Could you check a few things on this model? Use its own coordinates, in mm. A direction names the side the tool comes from. Round coordinates to 2 decimals unless told otherwise and drop trailing zeros. Write each loop counter-clockwise with the first axis right and the second up, starting at its lowest first coordinate (ties: lowest second). Pieces come first, ordered by that corner, then holes. Notation, with made-up numbers: (87.5, 9.25) -> (113.5, 9.25) arc R16 ccw to (113.5, 30.25) -> close; hole circle Ø8 at (67, -18). An arc over 180 degrees is marked (long way). Answer as CSV lines item,"result". Start each with the question number.
Q1. If we mould it in two halves opening along X, with no side actions, what happens to faces 1 (the flat face through (0, 6.1, -2)), 2 (the cylindrical face through (7.395, -2.028, 1.685)), 3 (the cylindrical face through (7.36, 1.99, -0.59))? For each: pulls with the +X half, pulls with the -X half, needs draft (parallel to the pull), parting line crosses it, or undercut.
Q2. For faces 4 (the flat face through (7.8, 3, -4.5)), 5 (the cylindrical face through (7.51, -2.03, 3.18)), 6 (the cylindrical face through (-4.956, 3.465, 5.072)), which set-ups out of +Z, -Z, +X, -X, +Y, -Y let a thin tool reach every point of the face, with its end or its side?
Q3. Imagine slicing it at B-B on y = -2.25. Please give me the cut outline in (x, z), and give its area (3 significant figures).
Q4. Imagine slicing it at D-D on x = 4.25. Please give me the cut outline in (y, z), and give its area (3 significant figures).
Q5. Imagine slicing it at C-C on y = 3.75. Please give me the cut outline in (x, z).
Q6. If I drill on line 1 (X direction, y = 0.6, z = -2.9); line 2 (Y direction, x = 4.5, z = 5.75); line 3 (Y direction, x = 5, z = -8), over which ranges is the centre line in solid material (lowest first)? Write a range as [from, to].
Q7. Will these pins go through, and if not, where does the flat tip stop? pin 1 Ø0.6 at (x, z) = (7.5, 3.5) entering from +Y; pin 2 Ø10 at (x, z) = (-4, 2) entering from -Y; pin 3 Ø1.6 at (x, z) = (-5, 6) entering from +Y.
Q8. Imagine slicing it at A-A on y = 1.5. Please give me the cut outline in (x, z).
from build123d import *

# Parameters (mm, degrees)
SKETCH1_W                = 17.5
SKETCH1_H                = 18
SKETCH1_R                = 0.4
BOSS_EXTRUDE1_DEPTH      = 1
SKETCH3_W                = 14
SKETCH3_H                = 17
SKETCH3_R                = 1
BOSS_EXTRUDE2_DEPTH      = 5
BOSS_EXTRUDE3_DEPTH      = 2
BOSS_EXTRUDE3_DEPTH_BACK = 5
SKETCH4_R                = 0.4
SKETCH5_R                = 5
BOSS_EXTRUDE4_DEPTH      = 0.1


with BuildPart() as part:
    # Sketch1 → Boss-Extrude1 (new body)
    with BuildSketch(Plane(origin=(0, 0, 0), x_dir=(1, 0, 0), z_dir=(0, 1, 0))):
        Rectangle(SKETCH1_W, SKETCH1_H)
        with Locations(Location((-7.95, -5.1, 0), (0, 0, 270))):
            Circle(SKETCH1_R, mode=Mode.SUBTRACT)
        with Locations(Location((-7.95, -3.1, 0), (0, 0, 270))):
            Circle(SKETCH1_R, mode=Mode.SUBTRACT)
        with Locations(Location((-7.95, -1.1, 0), (0, 0, 270))):
            Circle(SKETCH1_R, mode=Mode.SUBTRACT)
        with Locations(Location((-7.95, 0.9, 0), (0, 0, 270))):
            Circle(SKETCH1_R, mode=Mode.SUBTRACT)
        with Locations(Location((-7.95, 2.9, 0), (0, 0, 270))):
            Circle(SKETCH1_R, mode=Mode.SUBTRACT)
        with Locations(Location((-7.95, 4.9, 0), (0, 0, 270))):
            Circle(SKETCH1_R, mode=Mode.SUBTRACT)
    extrude(amount=BOSS_EXTRUDE1_DEPTH)

    # Sketch3 → Boss-Extrude2 (add)
    with BuildSketch(Plane(origin=(0, 1, 0), x_dir=(1, 0, 0), z_dir=(0, 1, 0))):
        Rectangle(SKETCH3_W, SKETCH3_H)
        with Locations(Location((-5, -6.071428571, 0), (0, 0, 270))):
            Circle(SKETCH3_R, mode=Mode.SUBTRACT)
        with Locations(Location((5, -6.071428571, 0), (0, 0, 270))):
            Circle(SKETCH3_R, mode=Mode.SUBTRACT)
    extrude(amount=BOSS_EXTRUDE2_DEPTH)

    # Sketch4 → Boss-Extrude3 (add, two sides: drawn at the far end of the back side and taken through both)
    with BuildSketch(Plane(origin=(0, 1, 0), x_dir=(1, 0, 0), z_dir=(0, 1, 0)).offset(-BOSS_EXTRUDE3_DEPTH_BACK)):
        with Locations(Location((7.75, 4.5, 0), (0, 0, 270))):
            Circle(SKETCH4_R)
        with Locations(Location((7.75, 2.5, 0), (0, 0, 270))):
            Circle(SKETCH4_R)
        with Locations(Location((7.75, 0.5, 0), (0, 0, 270))):
            Circle(SKETCH4_R)
        with Locations(Location((7.75, -1.5, 0), (0, 0, 270))):
            Circle(SKETCH4_R)
        with Locations(Location((7.75, -3.5, 0), (0, 0, 270))):
            Circle(SKETCH4_R)
    extrude(amount=BOSS_EXTRUDE3_DEPTH + BOSS_EXTRUDE3_DEPTH_BACK)

    # Sketch5 → Boss-Extrude4 (add)
    with BuildSketch(Plane(origin=(0, 6, 0), x_dir=(1, 0, 0), z_dir=(0, 1, 0))):
        with Locations(Location((0, 2, 0), (0, 0, 270))):
            Circle(SKETCH5_R)
    extrude(amount=BOSS_EXTRUDE4_DEPTH)


solid = part.part
Checks:
1,face 1,"needs draft"
1,face 2,"parting line crosses it"
1,face 3,"undercut"
2,face 4,"+Z, -Z, +X, +Y"
2,face 5,"-Y"
2,face 6,"+Y"
3,outline,"circle Ø0.8 at (7.75, -4.5); circle Ø0.8 at (7.75, -2.5); circle Ø0.8 at (7.75, -0.5); circle Ø0.8 at (7.75, 1.5); circle Ø0.8 at (7.75, 3.5)"
3,area,"2.51 mm^2"
4,outline,"(0, -9) -> (1, -9) -> (1, -8.5) -> (6, -8.5) -> (6, -4.63) -> (6.1, -4.63) -> (6.1, 0.63) -> (6, 0.63) -> (6, 5.41) -> (1, 5.41) -> (1, 6.73) -> (6, 6.73) -> (6, 8.5) -> (1, 8.5) -> (1, 9) -> (0, 9) -> close"
4,area,"96.9 mm^2"
5,outline,"(-7, -8.5) -> (7, -8.5) -> (7, 8.5) -> (-7, 8.5) -> close; hole circle Ø2 at (-5, 6.07); hole circle Ø2 at (5, 6.07)"
6,line 1,"[-8.75, -8.35], [-7.55, 8.75]"
6,line 2,"[0, 1]"
6,line 3,"[0, 6]"
7,pin 1,"y = 3"
7,pin 2,"y = 0"
7,pin 3,"y = 1"
8,outline,"(-7, -8.5) -> (7, -8.5) -> (7, 8.5) -> (-7, 8.5) -> close; circle Ø0.8 at (7.75, -4.5); circle Ø0.8 at (7.75, -2.5); circle Ø0.8 at (7.75, -0.5); circle Ø0.8 at (7.75, 1.5); circle Ø0.8 at (7.75, 3.5); hole circle Ø2 at (-5, 6.07); hole circle Ø2 at (5, 6.07)"
